from build123d import *

# Parameters (mm, degrees)
F1_W       = 10
F1_H       = 10
F2_DEPTH   = 10
F1_H_2     = 8
F1_W_2     = 20
F3_DEPTH   = 10
F5_DEPTH   = 15
F6_D       = 6
F6_DEPTH   = 20
F6_TIP     = 1.8025818571
F6_2_D     = 6
F6_2_DEPTH = 20
F6_2_TIP   = 1.8025818571
F6_3_D     = 6
F6_3_DEPTH = 20
F6_3_TIP   = 1.8025818571
F6_4_D     = 6
F6_4_DEPTH = 20
F6_4_TIP   = 1.8025818571
F6_5_D     = 6
F6_5_DEPTH = 20
F6_5_TIP   = 1.8025818571
F7_R       = 5
F7_2_R     = 5
F7_3_R     = 5
F7_4_R     = 5
F9_R       = 4.99999


# Not quite as in the source:
# - a fillet or chamfer is up to 0.001 mm smaller than in the source, because OpenCascade refuses the exact size


with BuildPart() as f2:
    # F1 (on Top) → F2 (new body)
    with BuildSketch(Plane.XY):
        with Locations((-20, -1.6993483007)):
            Rectangle(F1_W, F1_H)
    extrude(amount=F2_DEPTH)

    # F6
    with Locations(Plane(origin=(0, 0, 0), x_dir=(1, 0, 0), z_dir=(0, 0, -1))):
        with Locations((-20, 1.6993483007), (-5, 10.6993483007), (10, 1.6993483007), (10, 19.6993483007), (-20, 19.6993483007)):
            Hole(F6_D / 2, depth=F6_DEPTH)
            with Locations((0, 0, -(F6_DEPTH + F6_TIP / 2))):  # 118° drill point
                Cone(0, F6_D / 2, F6_TIP, mode=Mode.SUBTRACT)

    # F7
    f7_edges = [f2.edges().sort_by_distance(p)[0] for p in [
        (-25, 3.300652, 5),
    ]]
    fillet(f7_edges, radius=F7_R)


with BuildPart() as f2b:
    # F1 (on Top) → F2, piece 2 (new body)
    with BuildSketch(Plane.XY):
        with Locations((-20, -19.6993483007)):
            Rectangle(F1_W, F1_H)
    extrude(amount=F2_DEPTH)

    # F6#2
    with Locations(Plane(origin=(0, 0, 0), x_dir=(1, 0, 0), z_dir=(0, 0, -1))):
        with Locations((-20, 1.6993483007), (-5, 10.6993483007), (10, 1.6993483007), (10, 19.6993483007), (-20, 19.6993483007)):
            Hole(F6_2_D / 2, depth=F6_2_DEPTH)
            with Locations((0, 0, -(F6_2_DEPTH + F6_2_TIP / 2))):  # 118° drill point
                Cone(0, F6_2_D / 2, F6_2_TIP, mode=Mode.SUBTRACT)

    # F7#2
    f7_2_edges = [f2b.edges().sort_by_distance(p)[0] for p in [
        (-25, -24.699348, 5),
    ]]
    fillet(f7_2_edges, radius=F7_2_R)


with BuildPart() as f2c:
    # F1 (on Top) → F2, piece 3 (new body)
    with BuildSketch(Plane.XY):
        with Locations((10, -1.6993483007)):
            Rectangle(F1_W, F1_H)
    extrude(amount=F2_DEPTH)

    # F6#3
    with Locations(Plane(origin=(0, 0, 0), x_dir=(1, 0, 0), z_dir=(0, 0, -1))):
        with Locations((-20, 1.6993483007), (-5, 10.6993483007), (10, 1.6993483007), (10, 19.6993483007), (-20, 19.6993483007)):
            Hole(F6_3_D / 2, depth=F6_3_DEPTH)
            with Locations((0, 0, -(F6_3_DEPTH + F6_3_TIP / 2))):  # 118° drill point
                Cone(0, F6_3_D / 2, F6_3_TIP, mode=Mode.SUBTRACT)

    # F7#4
    f7_4_edges = [f2c.edges().sort_by_distance(p)[0] for p in [
        (15, 3.300652, 5),
    ]]
    fillet(f7_4_edges, radius=F7_4_R)


with BuildPart() as f2d:
    # F1 (on Top) → F2, piece 4 (new body)
    with BuildSketch(Plane.XY):
        with Locations((10, -19.6993483007)):
            Rectangle(F1_W, F1_H)
    extrude(amount=F2_DEPTH)

    # F6#4
    with Locations(Plane(origin=(0, 0, 0), x_dir=(1, 0, 0), z_dir=(0, 0, -1))):
        with Locations((-20, 1.6993483007), (-5, 10.6993483007), (10, 1.6993483007), (10, 19.6993483007), (-20, 19.6993483007)):
            Hole(F6_4_D / 2, depth=F6_4_DEPTH)
            with Locations((0, 0, -(F6_4_DEPTH + F6_4_TIP / 2))):  # 118° drill point
                Cone(0, F6_4_D / 2, F6_4_TIP, mode=Mode.SUBTRACT)

    # F7#3
    f7_3_edges = [f2d.edges().sort_by_distance(p)[0] for p in [
        (15, -24.699348, 5),
    ]]
    fillet(f7_3_edges, radius=F7_3_R)


with BuildPart() as f3:
    # F1 (on Top) → F3 (new body)
    with BuildSketch(Plane.XY):
        with Locations((-20, -10.6993483007)):
            Rectangle(F1_W, F1_H_2)
        with Locations((-5, -10.6993483007)):
            Rectangle(F1_W_2, F1_H_2)
        with Locations((10, -10.6993483007)):
            Rectangle(F1_W, F1_H_2)
    extrude(amount=F3_DEPTH)

    # F4 (on face) → F5 (cut)
    with BuildSketch(Plane(origin=(-25, 0, 0), x_dir=(0, -1, 0), z_dir=(-1, 0, 0))):
        with BuildLine():
            Line((14.6993483007, 10), (6.6993483007, 10))
            ThreePointArc((6.6993483007, 10), (10.6993483007, 8), (14.6993483007, 10))
        make_face()
    extrude(amount=-F5_DEPTH, mode=Mode.SUBTRACT)

    # F6#5
    with Locations(Plane(origin=(0, 0, 0), x_dir=(1, 0, 0), z_dir=(0, 0, -1))):
        with Locations((-20, 1.6993483007), (-5, 10.6993483007), (10, 1.6993483007), (10, 19.6993483007), (-20, 19.6993483007)):
            Hole(F6_5_D / 2, depth=F6_5_DEPTH)
            with Locations((0, 0, -(F6_5_DEPTH + F6_5_TIP / 2))):  # 118° drill point
                Cone(0, F6_5_D / 2, F6_5_TIP, mode=Mode.SUBTRACT)


with BuildPart() as f2_1:
    add(f2.part)

    # F8: union F2c, F3, F2b, F2d
    add(f2c.part)
    add(f3.part)
    add(f2b.part)
    add(f2d.part)

    # F9 (radius 5 in the source; OpenCascade refuses exactly that, so slightly less here)
    f9_edges = [f2_1.edges().sort_by_distance(p)[0] for p in [
        (-15, 3.300652, 5),
        (5, 3.300652, 5),
        (-15, -24.699348, 5),
        (5, -24.699348, 5),
        (-15, -14.699348, 5),
        (5, -14.699348, 5),
        (5, -6.699348, 5),
        (-15, -6.699348, 5),
    ]]
    fillet(f9_edges, radius=F9_R)


solid = f2_1.part
The model under review builds one solid part; all positions refer to its coordinate system, in mm. A direction names the side the tool comes from. Round coordinates to 2 decimals unless told otherwise and drop trailing zeros. Loops run counter-clockwise (first coordinate to the right, second up) from the corner with the lowest first, then second, coordinate; pieces in that order, holes last. Notation, with made-up numbers: M 39,89 L 94,89 A23 cw 94,114 Z; hole C 24.5,-13 d3. An arc over 180 degrees is marked long. Answer as CSV lines item,"result". Start each with the question number.
Item 1: Insertion check: P1, Ø8, axis at x = -20, y = -1.7, coming from the -Z side; P2, Ø3, axis at x = -3, z = 7.5, coming from the -Y side; P3, Ø2, axis at x = -12.5, z = 6.5, coming from the -Y side; P4, Ø3.5, axis at x = -20, y = -19.7, coming from the -Z side. Each pin has a flat end and moves straight along its axis. Give the tip position at first contact, or say it passes through.
Item 2: Consider section D-D (z = 7.5). State how many separate pieces and enclosed holes the cut face has, then the cut area to 3 significant figures.
Item 3: Wall thickness on line 1 (X direction, y = -19.5, z = 8.75); line 2 (Y direction, x = 10, z = 8); line 3 (X direction, y = -10.5, z = 3): over which ranges is each line inside the solid? List them lowest first. Write a range as [from, to].
Item 4: Consider section A-A (x = -5). Write out the cut boundary in (y, z).
Item 5: Consider section B-B (y = -15.5). Write out the cut boundary in (x, z).
Item 6: Mouldability with a two-part tool opening along X and no side actions: class faces 1 (the face through (13.5, -23.27, 5.07)), 2 (the face through (-17.79, -21.73, 5.07)), 3 (the face through (-23.57, 1.8, 5.07)), 4 (the face through (6.43, 1.8, 5.07)) as released by +X, released by -X, zero draft, split by the parting line, or undercut.
Item 7: Consider section C-C (x = 9.5). Write out the cut boundary in (y, z).
Item 8: For faces 5 (the face through (-17.6, -10.6, 8)), 6 (the face through (-5, -14.699, 5)), 7 (the face through (-16.5, 1.87, 5.07)), list the 3-axis set-ups (+Z, -Z, +X, -X, +Y, -Y) from which the entire face can be reached by the end or side of a thin tool; tool diameter is ignored.
Answer:
1,P1,"stops at z = 0"
1,P2,"stops at y = -14.7"
1,P3,"stops at y = -16.13"
1,P4,"passes through"
2,separate pieces,"1"
2,enclosed holes,"5"
2,area,"557 mm^2"
3,line 1,"x = [-25, -22.99], [-17.01, -15], [5, 7.01], [12.99, 15]"
3,line 2,"y = [-24.7, -22.7], [-16.7, -4.7], [1.3, 3.3]"
3,line 3,"x = [-25, -7.99], [-2.01, 15]"
4,outline,"M -14.7,0 L -13.7,0 L -13.7,10 L -14.7,10 Z; M -7.7,0 L -6.7,0 L -6.7,10 L -7.7,10 Z"
5,outline,"M -25,0 L -12.71,0 L -12.71,10 L -25,10 Z; M 2.71,0 L 15,0 L 15,10 L 2.71,10 Z"
6,face 1,"released by +X"
6,face 2,"undercut"
6,face 3,"released by -X"
6,face 4,"undercut"
7,outline,"M -24.67,0 L -22.66,0 L -22.66,10 L -24.67,10 Z; M -16.74,0 L -4.66,0 L -4.66,10 L -16.74,10 Z; M 1.26,0 L 3.28,0 L 3.28,10 L 1.26,10 Z"
8,face 5,"+Z, -X"
8,face 6,"+Z, -Z, -Y"
8,face 7,"+Z, -Z, +Y"
